from build123d import *

# Parameters (mm, degrees)
SKETCH_1_W          = 30
SKETCH_1_H          = 30
SKETCH_1_R          = 14
EXTRUDE_1_DEPTH     = 25
SKETCH_2_R          = 11.15
CUT_EXTRUDE_1_DEPTH = 42.833001327
SKETCH_3_R          = 1.363368529
CUT_EXTRUDE_2_DEPTH = 5


with BuildPart() as part:
    # 草图1 → 凸台-拉伸1 (new body)
    with BuildSketch(Plane.XY):
        Rectangle(SKETCH_1_W, SKETCH_1_H)
        Circle(SKETCH_1_R, mode=Mode.SUBTRACT)
    extrude(amount=EXTRUDE_1_DEPTH)

    # 草图2 → 切除-拉伸1 (cut, through all)
    with BuildSketch(Plane.ZY.offset(15)):
        with Locations((15, 0)):
            Circle(SKETCH_2_R)
    extrude(amount=-CUT_EXTRUDE_1_DEPTH, mode=Mode.SUBTRACT)

    # 草图3 → 切除-拉伸2 (cut)
    with BuildSketch(Plane(origin=(0, 0, 0), x_dir=(-1, 0, 0), z_dir=(0, 0, -1))):
        with Locations((12, 12)):
            Circle(SKETCH_3_R)
        with Locations((12, -12)):
            Circle(SKETCH_3_R)
        with Locations((-12, -12)):
            Circle(SKETCH_3_R)
        with Locations((-12, 12)):
            Circle(SKETCH_3_R)
    extrude(amount=-CUT_EXTRUDE_2_DEPTH, mode=Mode.SUBTRACT)


solid = part.part
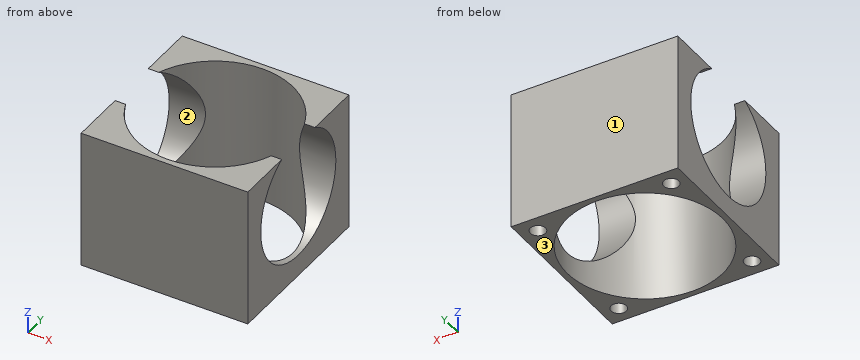
Work out the finished part from the listing and answer in its coordinate system (mm). Face numbers are marked on the shaded views. Give positions to 0.01 mm unless a question says otherwise; leave off trailing zeros. Loops run counter-clockwise (first coordinate to the right, second up) from the corner with the lowest first, then second, coordinate; pieces in that order, holes last. Notation, with made-up numbers: (-2.5, 10) - (1.5, 10) arc R28 ccw to (1.5, 33) - close; hole circle Ø10 at (15, -17). An arc over 180 degrees is marked (long way). Answer in a Markdown table with one row per item.
(1) Flat-ended cylindrical pins translate along their axes: pin 1 Ø17 at (x, y) = (0, 0) entering from +Z; pin 2 Ø0.8 at (x, y) = (11.5, -11.5) entering from -Z. Find the tip coordinate at first contact, or state that the pin passes through.
Results list:
| item | result |
|---|---|
| pin 1 | passes through |
| pin 2 | stops at z = 5 |
(2) For a pull along Y with two mould halves and no side action, classify the marked faces 1, 2 and 3 as pulls with the +Y half, pulls with the -Y half, needs draft (parallel to the pull), parting line crosses it, or undercut.
Results list:
| item | result |
|---|---|
| face 1 | pulls with the +Y half |
| face 2 | undercut |
| face 3 | needs draft |
(3) Section A-A (z = 15) is taken. Give the vertices of the cut face in (x, y).
Results list:
| item | result |
|---|---|
| outline | (-15, -15) - (15, -15) - (15, -11.15) - (8.47, -11.15) arc R14 cw to (-8.47, -11.15) - (-15, -11.15) - close; (-15, 11.15) - (-8.47, 11.15) arc R14 cw to (8.47, 11.15) - (15, 11.15) - (15, 15) - (-15, 15) - close |
(4) Section D-D (z = 3.25) is taken. Give the vertices of the cut face in (x, y), and give its area (3 significant figures).
Results list:
| item | result |
|---|---|
| outline | (-15, -15) - (15, -15) - (15, 15) - (-15, 15) - close; hole circle Ø28 at (0, 0); hole circle Ø2.73 at (-12, -12); hole circle Ø2.73 at (-12, 12); hole circle Ø2.73 at (12, -12); hole circle Ø2.73 at (12, 12) |
| area | 261 mm² |
(5) Consider L1, parallel to Y at x = 13.5, z = 5; L2, parallel to Y at x = 12, z = 3.6; L3, parallel to Y at x = 0, z = 11.25. Determine where each line is inside the solid, lowest interval first. Write a range as [from, to].
Results list:
| item | result |
|---|---|
| L1 | y = [-15, -4.93], [4.93, 15] |
| L2 | y = [-15, -13.36], [-10.64, -7.21], [7.21, 10.64], [13.36, 15] |
| L3 | y = [-15, -14], [14, 15] |
(6) Section C-C (y = -12.75) is taken. Give the vertices of the cut face in (x, z).
Results list:
| item | result |
|---|---|
| outline | (-15, 0) - (-13.14, 0) - (-13.14, 5) - (-10.86, 5) - (-10.86, 0) - (-5.78, 0) - (-5.78, 25) - (-15, 25) - close; (5.78, 0) - (10.86, 0) - (10.86, 5) - (13.14, 5) - (13.14, 0) - (15, 0) - (15, 25) - (5.78, 25) - close |
(7) Section B-B (x = 12) is taken. Give the vertices of the cut face in (y, z).
Results list:
| item | result |
|---|---|
| outline | (-15, 0) - (-13.36, 0) - (-13.36, 5) - (-10.64, 5) - (-10.64, 0) - (-7.21, 0) - (-7.21, 6.5) arc R11.15 cw to (-7.21, 23.5) - (-7.21, 25) - (-15, 25) - close; (7.21, 0) - (10.64, 0) - (10.64, 5) - (13.36, 5) - (13.36, 0) - (15, 0) - (15, 25) - (7.21, 25) - (7.21, 23.5) arc R11.15 cw to (7.21, 6.5) - close |
